```python
from build123d import *

# Parameters (mm, degrees)
SKETCH1_W           = 100
SKETCH1_H           = 100
BOSS_EXTRUDE1_DEPTH = 180
SKETCH2_R           = 34.257790197
BOSS_EXTRUDE2_DEPTH = 350
SKETCH3_W           = 152.006357392
SKETCH3_H           = 282.452416457
CUT_EXTRUDE2_DEPTH  = 400
CUT_EXTRUDE3_DEPTH  = 400
CUT_EXTRUDE4_DEPTH  = 400
CUT_EXTRUDE5_DEPTH  = 400
SKETCH7_W           = 160.159381639
SKETCH7_H           = 147.362276113
CUT_EXTRUDE6_DEPTH  = 400
SKETCH8_W           = 147.310744502
SKETCH8_H           = 162.038906966
CUT_EXTRUDE7_DEPTH  = 400
SKETCH9_R           = 31.847293423
CUT_EXTRUDE8_DEPTH  = 400


with BuildPart() as part:
    # Sketch1 → Boss-Extrude1 (new body)
    with BuildSketch(Plane(origin=(0, 0, 0), x_dir=(1, 0, 0), z_dir=(0, 1, 0))):
        with Locations((-50, 50)):
            Rectangle(SKETCH1_W, SKETCH1_H)
    extrude(amount=BOSS_EXTRUDE1_DEPTH)

    # Sketch2 → Boss-Extrude2 (add, symmetric)
    with BuildSketch(Plane(origin=(0, 180, 0), x_dir=(1, 0, 0), z_dir=(0, 1, 0))):
        with Locations(Location((-51.377291833, 49.076536384, 0), (0, 0, 270))):
            Circle(SKETCH2_R)
    extrude(amount=BOSS_EXTRUDE2_DEPTH, both=True)

    # Sketch3 → Cut-Extrude2 (cut)
    with BuildSketch(Plane(origin=(0, 0, 0), x_dir=(0, 0, -1), z_dir=(1, 0, 0))):
        with Locations((57.419900112, 502.274302507)):
            Rectangle(SKETCH3_W, SKETCH3_H)
    extrude(amount=-CUT_EXTRUDE2_DEPTH, mode=Mode.SUBTRACT)

    # Sketch4 → Cut-Extrude3 (cut)
    with BuildSketch(Plane(origin=(0, 0, 0), x_dir=(0, 0, -1), z_dir=(1, 0, 0))):
        Polygon((12.981970869, 0), (-8.994244796, 25.828096003), (-18.564506014, -15.259465835), align=None)
        Polygon((85.072517936, -1.448103984), (109.237639161, 19.113145112), (115.920034239, -3.267382694), align=None)
        Polygon((12.981970869, 180), (-8.994244796, 148.537596011), (-15.418178585, 193.219274892), align=None)
        Polygon((85.072517936, 181.854312784), (103.841225373, 159.795920888), (106.132549481, 198.647393934), align=None)
    extrude(amount=-CUT_EXTRUDE3_DEPTH, mode=Mode.SUBTRACT)

    # Sketch5 → Cut-Extrude4 (cut)
    with BuildSketch(Plane.XY):
        Polygon((-85.623287335, 0), (-106.370377984, 21.426392531), (-122.288861874, 3.209259887), (-93.526345261, -19.884701759), align=None)
        Polygon((-15.694988751, 0), (0, 15.257385304), (12.122677088, 15.257385304), (10.563067769, -19.884701759), align=None)
        Polygon((-87.166490339, 180.248071029), (-106.370377984, 151.29108453), (-117.705469457, 200.501115102), align=None)
        Polygon((-15.694988751, 180.248071029), (7.833767065, 153.279557508), (0, 193.941208308), align=None)
    extrude(amount=-CUT_EXTRUDE4_DEPTH, mode=Mode.SUBTRACT)

    # Sketch6 → Cut-Extrude5 (cut)
    with BuildSketch(Plane(origin=(0, 180, 0), x_dir=(1, 0, 0), z_dir=(0, 1, 0))):
        Polygon((-112.386997555, 28.400400964), (-64.261264503, -10.212759359), (-84.406366528, -15.51192827), (-124.649689542, -15.51192827), align=None)
        Polygon((-97.065537028, 135.861756084), (-119.37552445, 77.792688888), (-118.043343626, 64.347606737), (-66.428694172, 110.575168787), align=None)
        Polygon((-24.69640689, -21.815840769), (11.092108798, -8.97361337), (17.428316417, 32.393768119), (-38.531576846, -11.139157378), align=None)
        Polygon((-17.445484601, 140.804394854), (35.417473102, 107.262520599), (9.305452855, 72.996438725), (-31.724385352, 103.625272537), align=None)
    extrude(amount=-CUT_EXTRUDE5_DEPTH, mode=Mode.SUBTRACT)

    # Sketch7 → Cut-Extrude6 (cut)
    with BuildSketch(Plane.XY):
        with Locations((-66.123258915, -136.36252694)):
            Rectangle(SKETCH7_W, SKETCH7_H)
    extrude(amount=-CUT_EXTRUDE6_DEPTH, mode=Mode.SUBTRACT)

    # Sketch8 → Cut-Extrude7 (cut)
    with BuildSketch(Plane.XY):
        with Locations((-53.541153336, 332.448287589)):
            Rectangle(SKETCH8_W, SKETCH8_H)
    extrude(amount=-CUT_EXTRUDE7_DEPTH, mode=Mode.SUBTRACT)

    # Sketch9 → Cut-Extrude8 (cut)
    with BuildSketch(Plane(origin=(0, 251.428834106, 0), x_dir=(1, 0, 0), z_dir=(0, 1, 0))):
        with Locations(Location((-50.808993157, 49.032036374, 0), (0, 0, 270))):
            Circle(SKETCH9_R)
    extrude(amount=-CUT_EXTRUDE8_DEPTH, mode=Mode.SUBTRACT)


solid = part.part
```
Source: CAD feature listing. Evaluate the final solid. Frame: model axes, mm. A direction names the side the tool comes from. Coordinates: 2 decimals unless noted, no trailing zeros. Loops run counter-clockwise (first coordinate to the right, second up) from the corner with the lowest first, then second, coordinate; pieces in that order, holes last. Notation, with made-up numbers: M -4.75,67 L 6.25,67 A22 cw 6.25,80 Z; hole C 5,-35.5 d7. An arc over 180 degrees is marked long. Use a Markdown table: item, result. Add a question column.
Q1. Material intervals for L1, parallel to X at y = 68, z = -28; L2, parallel to Y at x = -76.5, z = -13.5; L3, parallel to X at y = -29.5, z = -62.5, sorted ascending.
Q2. Section query B-B, the plane y = 100.5. Return loops of the section in (x, z).
Q3. Access query for faces 5 (the cylindrical face through (-84.82, 216.21, -56.5)), 6 (the flat face through (-25, 0, -72)), 7 (the flat face through (-82, 251.429, -57)). Directions: +Z, -Z, +X, -X, +Y, -Y. A direction counts if a zero-diameter tool reaches every point of the face in a straight line with its end or side. Return the directions, or none.
Q4. Draft query along X for faces 1 (the flat face through (-82, -62.681, -57)), 2 (the cylindrical face through (-70.188, 96.572, -74.305)), 3 (the flat face through (-88.656, 91.164, -9.36)), 4 (the flat face through (-7.848, 171.253, -49.063)). Return one class per face: pulls with the +X half, pulls with the -X half, needs draft (parallel to the pull), parting line crosses it, or undercut.
Q5. Section query C-C, the plane z = -33.5. Return loops of the section in (x, y).
Q6. Section query A-A, the plane z = -66.5. Return loops of the section in (x, y), and give its area (3 significant figures).
Q7. First-contact query: pin 1 (8 mm diameter, centred on y = -20, z = -79, fed in from -X); pin 2 (6 mm diameter, centred on x = -78, y = -30.5, fed in from +Z); pin 3 (1.5 mm diameter, centred on y = 174, z = -40.5, fed in from +X). Flat tips, straight axial feed; report the tip coordinate or a pass-through.
Q8. Section query D-D, the plane x = -93. Return loops of the section in (y, z).
Result:
| question | item | result |
|---|---|---|
| 1 | L1 | x = -100 to -74.72, -26.89 to 0 |
| 1 | L2 | y = 0 to 180 |
| 1 | L3 | x = -82.9 to -79.67, -21.95 to -19.86 |
| 2 | outline | M -100,-80.51 L -78.24,-100 L -26.87,-100 L 0,-79.94 L 0,-18.84 L -24.21,0 L -76.99,0 L -100,-18.46 Z; hole C -50.81,-49.03 d63.69 |
| 3 | face 5 | +Y |
| 3 | face 6 | -Y |
| 3 | face 7 | +Z, -Z, +X, -X, +Y |
| 4 | face 1 | needs draft |
| 4 | face 2 | undercut |
| 4 | face 3 | pulls with the -X half |
| 4 | face 4 | pulls with the +X half |
| 5 | outline | M -100,14.85 L -85.62,0 L -81.89,0 L -81.89,-62.68 L -78.61,-62.68 L -78.61,251.43 L -81.89,251.43 L -81.89,180 L -87.33,180 L -100,160.9 Z; M -23.01,-62.68 L -20.87,-62.68 L -20.87,0 L -15.69,0 L 0,15.26 L 0,162.26 L -15.48,180 L -20.87,180 L -20.87,251.43 L -23.01,251.43 Z |
| 6 | outline | M -100,14.85 L -85.62,0 L -80.87,0 L -80.87,-62.68 L -77.44,-62.68 L -77.44,251.43 L -80.87,251.43 L -80.87,180 L -87.33,180 L -100,160.9 Z; M -24.18,-62.68 L -21.88,-62.68 L -21.88,0 L -15.69,0 L 0,15.26 L 0,162.26 L -15.48,180 L -21.88,180 L -21.88,251.43 L -24.18,251.43 Z |
| 6 | area | 8,700 mm2 |
| 7 | pin 1 | stops at x = -73.77 |
| 7 | pin 2 | stops at z = -24.27 |
| 7 | pin 3 | stops at x = -9.59 |
| 8 | outline | M 7.62,-86.78 L 171.45,-86.78 L 171.45,-12.85 L 7.62,-12.85 Z |
